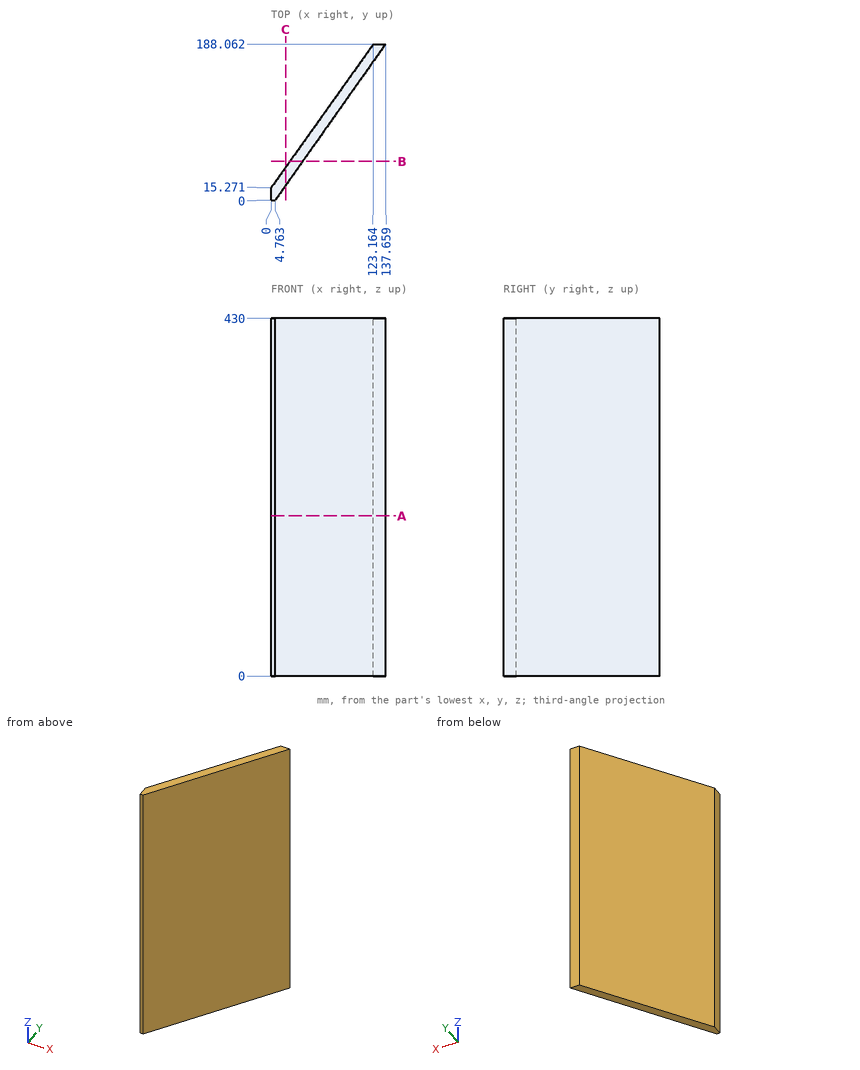
Source: three-view drawing plus pictorial views. Frame: mm from the lowest corner of the part. Coordinates: 2 decimals unless noted, no trailing zeros. Loops run counter-clockwise (first coordinate to the right, second up) from the corner with the lowest first, then second, coordinate; pieces in that order, holes last. Notation, with made-up numbers: (21.25, -9.5) -> (29.25, -9.5) arc R15 ccw to (29.25, 4.5) -> close; hole circle Ø10 at (48, -36.5). An arc over 180 degrees is marked (long way). Write each question's results on one line, items separated by ' | '. Start each with the question number.
Q1. Section B-B, the plane y = 47. Return the cut outline in (x, z) (1 decimal).
Q2. Pin query (flat end, axial travel): pin 1 (8 mm diameter, centred on y = 36, z = 336.5, fed in from -X) (1 decimal); pin 2 (8 mm diameter, centred on y = 163.5, z = 184.5, fed in from -X) (1 decimal); pin 3 (4 mm diameter, centred on x = 21.5, z = 269, fed in from +Y). Return the tip coordinate at first contact, or that it passes through.
Q3. Section C-C, the plane x = 17.5. Return the cut outline in (y, z) (1 decimal), plus the area to 3 significant figures.
Q4. Section A-A, the plane z = 192.5. Return the cut outline in (x, y) (1 decimal).
Q5. Ray query, line 1 (X direction, y = 42, z = 71.5); line 2 (Y direction, x = 18, z = 316) (1 decimal); line 3 (X direction, y = 121.5, z = 388). Return the intervals inside material, ascending. Write a range as from..to.
Found:
1) outline: (22.6, 0) -> (38, 0) -> (38, 430) -> (22.6, 430) -> close
2) pin 1: x = 11.9 | pin 2: x = 102.8 | pin 3: y = 48.24
3) outline: (18, 0) -> (39.8, 0) -> (39.8, 430) -> (18, 430) -> close | area: 9,370 mm2
4) outline: (0, 0) -> (4.8, 0) -> (137.7, 188.1) -> (123.2, 188.1) -> (0, 15.3) -> close
5) line 1: 19.05..34.44 | line 2: 18.7..40.5 | line 3: 75.72..90.62
